The listing builds one solid part. Answer for the finished solid, in the listing's coordinates (mm). Face numbers are marked on the shaded views. A direction names the side the tool comes from. Give positions to 0.01 mm unless a question says otherwise; leave off trailing zeros. Order: outer loops, then holes, each group sorted by start corner. A loop starts at its lowest first (then second) coordinate and runs counter-clockwise, first axis right, second up.
```python
from build123d import *

# Parameters (mm, degrees)
BOSS_EXTRUDE1_DEPTH = 50
CUT_EXTRUDE1_DEPTH  = 35
CUT_EXTRUDE2_DEPTH  = 15


with BuildPart() as part:
    # Sketch1 → Boss-Extrude1 (new body)
    with BuildSketch(Plane.XY):
        Polygon((0, 30), (0, 0), (30, 10), (30, 40), align=None)
        Polygon((30, 40), (30, 10), (60, 20), (60, 50), align=None)
        Polygon((30, 10), (0, 0), (60, 0), (60, 20), align=None)
    extrude(amount=BOSS_EXTRUDE1_DEPTH)

    # Sketch2 → Cut-Extrude1 (cut)
    with BuildSketch(Plane.XY.offset(50)):
        Polygon((30, 10), (30, 40), (0, 30), (0, 0), align=None)
    extrude(amount=-CUT_EXTRUDE1_DEPTH, mode=Mode.SUBTRACT)

    # Sketch3 → Cut-Extrude2 (cut)
    with BuildSketch(Plane.XY.offset(50)):
        Polygon((30, 40), (60, 50), (60, 20), (30, 10), align=None)
    extrude(amount=-CUT_EXTRUDE2_DEPTH, mode=Mode.SUBTRACT)


solid = part.part
```
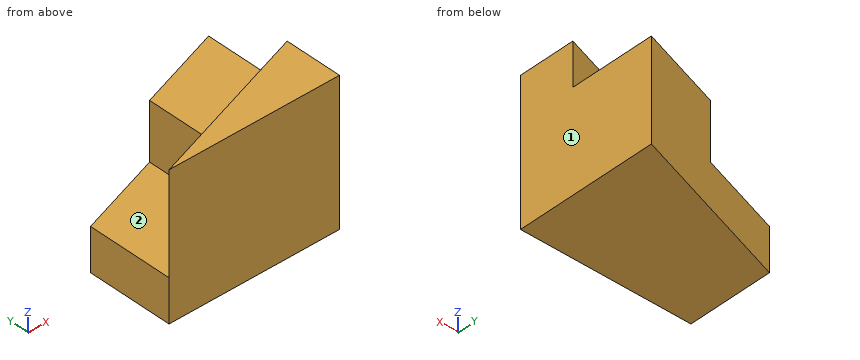
1) Straight lines are drawn through the part: probe 1 along Z at (x, y) = (41, 32); probe 2 along Z at (x, y) = (14, 24); probe 3 along X at (y, z) = (25.5, 17). For each, find the intervals that lie inside material, in ascending order.
Geometry says:
probe 1: z = 0 to 35
probe 2: z = 0 to 15
probe 3: x = 30 to 60
2) Find section B-B (x = 34.5). Write down the section's boundary in (y, z).
Geometry says:
outline: (0, 0) - (41.5, 0) - (41.5, 35) - (11.5, 35) - (11.5, 50) - (0, 50) - close
3) A tool of negligible diameter and unlimited length cuts with its end or side. For the marked faces 1 and 2, from which of +Z, -Z, +X, -X, +Y, -Y can it reach the whole face along a straight path? Write none if from no direction.
Geometry says:
face 1: +Z, -Z, +X, +Y, -Y
face 2: +Z, -X, +Y
4) Find section D-D (z = 10.5). Write down the section's boundary in (x, y), then the cut area to 3 significant figures.
Geometry says:
outline: (0, 0) - (60, 0) - (60, 50) - (0, 30) - close
area: 2,400 mm2
5) Find section C-C (z = 31). Write down the section's boundary in (x, y), then the cut area to 3 significant figures.
Geometry says:
outline: (0, 0) - (60, 0) - (60, 50) - (30, 40) - (30, 10) - close
area: 1,500 mm2
6) Find section A-A (y = 9). Write down the section's boundary in (x, z), then the cut area to 4 significant figures.
Geometry says:
outline: (0, 0) - (60, 0) - (60, 50) - (27, 50) - (27, 15) - (0, 15) - close
area: 2,055 mm2
7) Given P1, Ø1, axis at x = 21, y = 23, coming from the +Z side; P2, Ø5, axis at x = 46, z = 8.5, coming from the +Y side; P3, Ø1.5, axis at y = 16, z = 27, coming from the -X side, each flat-ended and moving along its own axis, determine where each tip first touches the part or whether it passes through.
Geometry says:
P1: stops at z = 15
P2: stops at y = 46.17
P3: stops at x = 30
